from build123d import *

# Parameters (mm, degrees)
F0_W          = 203.2
F0_H          = 101.6
F1_DEPTH      = 20.574
F1_TAPER      = 10
F1_DEPTH_BACK = 19.812
F1_TAPER_BACK = -15
F2_T          = -7.62
F3_T1_DEPTH   = 238.5707586616
F3_T3_DEPTH   = 136.9707586616


# Not quite as in the source:
# - a fillet or chamfer that OpenCascade refuses, or shapes differently, is made with other operations: its cross-section is extruded or revolved along the edge and cut away or added


with BuildPart() as f1:
    # F0 (on Top) → F1 (new body, two sides)
    with BuildSketch(Plane.XY) as f1_sk:
        with Locations((0.4991553724, 21.9660702551)):
            Rectangle(F0_W, F0_H)
    extrude(amount=F1_DEPTH, taper=F1_TAPER)
    extrude(f1_sk.sketch, amount=-F1_DEPTH_BACK, taper=F1_TAPER_BACK)

    # F2
    f2_openings = [f1.faces().sort_by_distance(p)[0] for p in [
        (0.499155, 21.96607, 20.574),
        (0.499155, 21.96607, -19.812),
    ]]
    offset(amount=F2_T, openings=f2_openings, kind=Kind.INTERSECTION)

    # F3: fillet of radius 10.16 on 4 edges, made by hand

    # F3_s2 → F3_t1 (cut)
    with BuildSketch(Plane.YZ.offset(-118.7862239584)):
        with BuildLine():
            ThreePointArc((70.6187134719, 12.1782654851), (67.1437888157, 18.1970115421), (60.6130667013, 20.574))
            Line((60.6130667013, 20.574), (69.138318954, 20.574))
            Line((69.138318954, 20.574), (70.6187134719, 12.1782654851))
        make_face()
        with BuildLine():
            ThreePointArc((-26.6865729616, 12.1782654851), (-23.2116483054, 18.1970115421), (-16.680926191, 20.574))
            Line((-16.680926191, 20.574), (-25.2061784438, 20.574))
            Line((-25.2061784438, 20.574), (-26.6865729616, 12.1782654851))
        make_face()
    extrude(amount=F3_T1_DEPTH, mode=Mode.SUBTRACT)

    # F3_s4 → F3_t3 (cut)
    with BuildSketch(Plane.XZ.offset(-90.4514495859)):
        with BuildLine():
            ThreePointArc((99.9517985891, 12.1782654851), (96.4768739329, 18.1970115421), (89.9461518185, 20.574))
            Line((89.9461518185, 20.574), (98.4714040713, 20.574))
            Line((98.4714040713, 20.574), (99.9517985891, 12.1782654851))
        make_face()
        with BuildLine():
            ThreePointArc((-98.9534878444, 12.1782654851), (-95.4785631882, 18.1970115421), (-88.9478410738, 20.574))
            Line((-88.9478410738, 20.574), (-97.4730933265, 20.574))
            Line((-97.4730933265, 20.574), (-98.9534878444, 12.1782654851))
        make_face()
    extrude(amount=F3_T3_DEPTH, mode=Mode.SUBTRACT)


solid = f1.part
Read the model definition and answer for the solid it produces. Units are mm, in the model's axes. A direction names the side the tool comes from. Give positions to 0.01 mm unless a question says otherwise; leave off trailing zeros. Write each loop counter-clockwise with the first axis right and the second up, starting at its lowest first coordinate (ties: lowest second). Pieces come first, ordered by that corner, then holes. Notation, with made-up numbers: (-14, 36) - (9, 36) arc R25 cw to (9, 49) - close; hole circle Ø10 at (-4.5, -36.5). An arc over 180 degrees is marked (long way). Answer in a Markdown table with one row per item. Add a question column.
Item 1: A tool of negligible diameter and unlimited length cuts with its end or side. For faces 1 (the face through (92.723, 22.573, 9.291)), 2 (the face through (-0.89, -23.58, 17.87)), from which of +Z, -Z, +X, -X, +Y, -Y can it reach the whole face along a straight path? Write none if from no direction.
Item 2: Find the intervals of material crossed by L1, parallel to Y at x = -44, z = -16; L2, parallel to X at y = 2.5, z = -17; L3, parallel to X at y = -16.5, z = -6.5, in increasing order.
Item 3: Flat-ended cylindrical pins translate along their axes: P1, Ø6, axis at y = 62.5, z = 13, coming from the +X side; P2, Ø5, axis at y = -6.5, z = -4, coming from the -X side; P3, Ø2, axis at x = 24.5, z = 8, coming from the -Y side. Find the tip coordinate at first contact, or state that the pin passes through.
Item 4: Section A-A, the plane z = 3 is taken. Write down the section's boundary in (x, y), and give its area (3 significant figures).
Item 5: Determine the mould class of faces 3 (the face through (-100.042, 21.255, 6.004)), 4 (the face through (14, 71, -19.812)), 5 (the face through (-0.887, -23.855, -10.859)), 6 (the face through (101.04, 22.68, 6)) for opening direction X: pulls with the +X half, pulls with the -X half, needs draft (parallel to the pull), parting line crosses it, or undercut.
Recorded:
| question | item | result |
|---|---|---|
| 1 | face 1 | -Z |
| 1 | face 2 | +Z, +X, -X, -Y |
| 2 | L1 | y = -33.12 to -25.23, 69.16 to 77.05 |
| 2 | L2 | x = -105.66 to -97.77, 98.77 to 106.65 |
| 2 | L3 | x = -102.84 to -94.95, 95.95 to 103.84 |
| 3 | P1 | stops at x = 100.34 |
| 3 | P2 | stops at x = -102.84 |
| 3 | P3 | stops at y = -27.6 |
| 4 | outline | (-100.57, -28.3) - (101.57, -28.3) - (101.57, 72.24) - (-100.57, 72.24) - close; hole (-92.83, -20.57) - (93.83, -20.57) - (93.83, 64.5) - (-92.83, 64.5) - close |
| 4 | area | 4,440 mm2 |
| 5 | face 3 | pulls with the -X half |
| 5 | face 4 | needs draft |
| 5 | face 5 | undercut |
| 5 | face 6 | pulls with the +X half |
